```python
from build123d import *

# Parameters (mm, degrees)
F0_R     = 1.3589
F0_R_2   = 3.81
F1_DEPTH = 1.5875
F2_R     = 12.7


with BuildPart() as f1:
    # F0 (on Top) → F1 (new body)
    with BuildSketch(Plane.XY):
        with BuildLine():
            Line((0, 12.7), (0, 0))
            Line((0, 0), (165.1, 0))
            Line((165.1, 0), (165.1, 25.4))
            Line((165.1, 25.4), (165.1, 165.1))
            Line((165.1, 165.1), (164.819603, 165.1))
            Line((164.819603, 165.1), (152.119603, 165.099742))
            ThreePointArc((152.119603, 165.099742), (44.537837, 120.363893), (0, 12.7))
        make_face()
        with Locations((142.61465, 12.7)):
            Circle(F0_R, mode=Mode.SUBTRACT)
        with Locations((152.4, 2.91465)):
            Circle(F0_R, mode=Mode.SUBTRACT)
        with Locations((145.480713, 5.780713)):
            Circle(F0_R, mode=Mode.SUBTRACT)
        with Locations((159.319287, 5.780713)):
            Circle(F0_R, mode=Mode.SUBTRACT)
        with Locations((152.4, 12.7)):
            Circle(F0_R_2, mode=Mode.SUBTRACT)
        with Locations((145.480713, 19.619287)):
            Circle(F0_R, mode=Mode.SUBTRACT)
        with Locations((162.18535, 12.7)):
            Circle(F0_R, mode=Mode.SUBTRACT)
        with Locations((159.319287, 19.619287)):
            Circle(F0_R, mode=Mode.SUBTRACT)
        with Locations((152.4, 22.48535)):
            Circle(F0_R, mode=Mode.SUBTRACT)
        with BuildLine():
            ThreePointArc((31.783426, 30.48), (66.189541, 98.910459), (134.62, 133.316574))
            Line((134.62, 133.316574), (134.62, 30.48))
            Line((134.62, 30.48), (31.783426, 30.48))
        make_face(mode=Mode.SUBTRACT)
    extrude(amount=F1_DEPTH)

    # F2
    f2_edges = [f1.edges().sort_by_distance(p)[0] for p in [
        (165.1, 0, 0.79375),
    ]]
    fillet(f2_edges, radius=F2_R)


solid = f1.part
```
Check sheet for the modelled part. Datum: model origin and axes. Units: mm. Round coordinates to 2 decimals unless told otherwise and drop trailing zeros. Loops run counter-clockwise (first coordinate to the right, second up) from the corner with the lowest first, then second, coordinate; pieces in that order, holes last. Notation, with made-up numbers: M -7,3 L 26,3 A16 ccw 26,12 Z; hole C 82,-15.75 d11. An arc over 180 degrees is marked long. Answer as a JSON object with one key per item and string values.
1. Section check B-B (z = 1.3). State how many separate pieces and enclosed holes the cut face has, plus the area to 3 significant figures.
Reply:
{"separate pieces": "1", "enclosed holes": "10", "area": "14,500 mm²"}
2. Scan lines: line 1 (Y direction, x = 39.5, z = 0.5); line 2 (X direction, y = 49.5, z = 0.2); line 3 (Y direction, x = 142.5, z = 1.4). Record each from-to range of solid material in increasing order.
Reply:
{"line 1": "y = 0 to 30.48, 58.72 to 115.07", "line 2": "x = 4.51 to 36.17, 134.62 to 165.1", "line 3": "y = 0 to 11.35, 14.05 to 164.78"}
3. Mould release check, pull along Y, two halves, no side actions. Record for faces 1 (the cylindrical face through (148.594, 12.868, 0.783)), 2 (the cylindrical face through (65.422, 98.136, 0.783)), 3 (the cylindrical face through (161.28, 3.62, 0.8)), 4 (the flat face through (63, 102, 0)): pulls with the +Y half, pulls with the -Y half, needs draft (parallel to the pull), parting line crosses it, or undercut.
Reply:
{"face 1": "undercut", "face 2": "undercut", "face 3": "pulls with the -Y half", "face 4": "needs draft"}
4. Section check A-A (x = 36.5). Record the boundary of the cut face in (y, z).
Reply:
{"outline": "M 0,0 L 30.48,0 L 30.48,1.59 L 0,1.59 Z; M 50.54,0 L 111.66,0 L 111.66,1.59 L 50.54,1.59 Z"}
5. Gauge pin test, flat ends, axial feed: P1, Ø0.8, axis at y = 77.5, z = 0.5, coming from the -X side; P2, Ø0.5, axis at x = 107, z = 1, coming from the +Y side. Record the tip position at first contact, or that the pin passes through.
Reply:
{"P1": "stops at x = 14.28", "P2": "stops at y = 158.26"}
6. Section check C-C (y = 80.5). Record the boundary of the cut face in (x, z).
Reply:
{"outline": "M 15.91,0 L 51.07,0 L 51.07,1.59 L 15.91,1.59 Z; M 134.62,0 L 165.1,0 L 165.1,1.59 L 134.62,1.59 Z"}
